Can you work these out from the model? Positions are in its coordinate system, mm. A direction names the side the tool comes from. Give positions to 0.01 mm unless a question says otherwise; leave off trailing zeros. Order: outer loops, then holes, each group sorted by start corner. A loop starts at its lowest first (then second) coordinate and runs counter-clockwise, first axis right, second up.
```python
from build123d import *

# Parameters (mm, degrees)
BOSS_EXTRUDE1_DEPTH = 5.715
CUT_EXTRUDE1_DEPTH  = 257.4305006


with BuildPart() as part:
    # Model → Boss-Extrude1 (new body)
    with BuildSketch(Plane.XY):
        Polygon((861.0219, 23.2006394), (866.70388, 23.2006394), (866.70388, 28.91536), (878.13388, 28.91536), (878.13388, 23.2006394), (889.56896, 23.2006394), (889.56896, 28.91536), (900.99388, 28.91536), (900.99388, 23.2006394), (912.42896, 23.2006394), (912.42896, 28.91536), (923.85388, 28.91536), (923.85388, 23.2006394), (935.28388, 23.2006394), (935.28388, 28.91536), (946.71896, 28.91536), (946.71896, 23.2006394), (958.11594, 23.2006394), (958.11594, 279.63114), (946.71896, 279.63114), (946.71896, 273.91614), (935.28388, 273.91614), (935.28388, 279.63114), (923.85388, 279.63114), (923.85388, 273.91614), (912.42896, 273.91614), (912.42896, 279.63114), (900.99388, 279.63114), (900.99388, 273.91614), (889.56896, 273.91614), (889.56896, 279.63114), (878.13388, 279.63114), (878.13388, 273.91614), (866.70388, 273.91614), (866.70388, 279.63114), (855.3069, 279.63114), (855.3069, 23.2006394), align=None)
    extrude(amount=BOSS_EXTRUDE1_DEPTH)

    # Sketch1 → Cut-Extrude1 (cut, through all)
    with BuildSketch(Plane.XZ.offset(-23.2006394)):
        Polygon((855.3069, 2.8575), (858.1644, 5.715), (855.3069, 5.715), align=None)
        Polygon((958.11594, 2.8575), (955.25844, 0), (958.11594, 0), align=None)
    extrude(amount=-CUT_EXTRUDE1_DEPTH, mode=Mode.SUBTRACT)


solid = part.part
```
1) I'm going to push flat-ended pins straight in: pin 1 Ø1.7 at (x, z) = (941.5, 2.5) entering from -Y; pin 2 Ø1.7 at (y, z) = (25.5, 4) entering from -X. Where does each tip first touch, or does it pass through?
2) We'd pull the mould along X, two halves only. Please class faces 1 (the face through (941, 28.915, 3)), 2 (the face through (884, 279.631, 3)): +X half, -X half, draft (parallel to the pull), parting line (faces both ways), or undercut.
3) Which directions (+Z, -Z, +X, -X, +Y, -Y) give clear straight access to the entire face, cutting with the end or side of a thin tool? Please do faces 3 (the face through (866.704, 277, 3)), 4 (the face through (889.569, 26, 3)), 5 (the face through (907, 279.631, 3)).
4) If I drill on line 1 (Y direction, x = 875, z = 1.65); line 2 (X direction, y = 210.5, z = 2.6); line 3 (X direction, y = 174, z = 0.85), over which ranges is the centre line in solid material (lowest first)?
5) Suppose I cut it at A-A (x = 873.5). Please give me the cut outline in (y, z) (3 decimals).
Results:
1. pin 1: stops at y = 28.92
1. pin 2: stops at x = 855.6
2. face 1: undercut
2. face 2: draft
3. face 3: +Z, -Z, +Y
3. face 4: +Z, -Z, -Y
3. face 5: +Z, -Z, +X, -X, +Y
4. line 1: y = 28.92 to 273.92
4. line 2: x = 855.31 to 957.86
4. line 3: x = 855.31 to 956.11
5. outline: (28.915, 0) - (273.916, 0) - (273.916, 5.715) - (28.915, 5.715) - close
